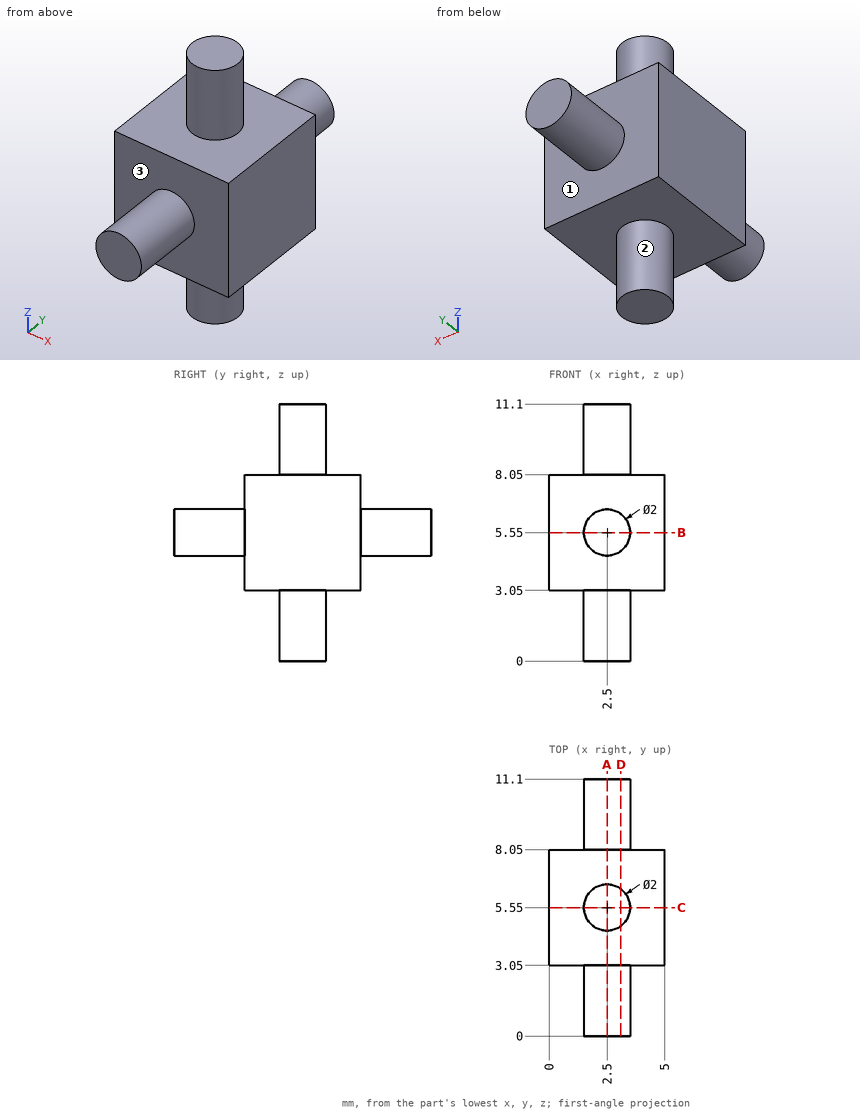
Drawing for the job (mm, zero at the part's lowest x, y, z). A direction names the side the tool comes from. Give positions to 0.01 mm unless a question says otherwise; leave off trailing zeros. Write each loop counter-clockwise with the first axis right and the second up, starting at its lowest first coordinate (ties: lowest second). Pieces come first, ordered by that corner, then holes. Notation, with made-up numbers: M -18,48 L -1,48 A15 cw -1,63 Z; hole C 6.5,42 d2. An arc over 180 degrees is marked long. Return JSON: item names as keys, results as strings. Group by question number.
(1) 3-axis set-ups, long thin cutter, end or side, ignore diameter. For the marked faces 1, 2 and 3: which of +Z, -Z, +X, -X, +Y, -Y reach the whole face in a straight line?
(2) Band-saw the part on B-B (z = 5.55). Give the cut face in (x, y).
(3) Band-saw the part on D-D (x = 3.1). Give the cut face in (y, z), and give its area (3 significant figures).
(4) Flat gauge pins, fed straight in: pin 1 Ø2.5 at (x, z) = (2, 5.5) entering from -Y; pin 2 Ø1 at (y, z) = (9, 2.5) entering from +X. Where does each tip first touch, or does it go through?
(5) Drill centre lines: L1, parallel to Y at x = 2.75, z = 7.75; L2, parallel to Z at x = 2.55, y = 1.75. Where is each one in solid material? Low to high. Write a range as [from, to].
(6) Band-saw the part on A-A (x = 2.5). Give the cut face in (y, z), and give its area (3 significant figures).
Entries:
{
 "1": {"face 1": "+Y", "face 2": "-Z", "face 3": "-Y"},
 "2": {"outline": "M 0,3.05 L 1.5,3.05 L 1.5,0 L 3.5,0 L 3.5,3.05 L 5,3.05 L 5,8.05 L 3.5,8.05 L 3.5,11.1 L 1.5,11.1 L 1.5,8.05 L 0,8.05 Z"},
 "3": {"outline": "M 0,4.75 L 3.05,4.75 L 3.05,3.05 L 4.75,3.05 L 4.75,0 L 6.35,0 L 6.35,3.05 L 8.05,3.05 L 8.05,4.75 L 11.1,4.75 L 11.1,6.35 L 8.05,6.35 L 8.05,8.05 L 6.35,8.05 L 6.35,11.1 L 4.75,11.1 L 4.75,8.05 L 3.05,8.05 L 3.05,6.35 L 0,6.35 Z", "area": "44.5 mm^2"},
 "4": {"pin 1": "stops at y = 0", "pin 2": "passes through"},
 "5": {"L1": "y = [3.05, 8.05]", "L2": "z = [4.55, 6.55]"},
 "6": {"outline": "M 0,4.55 L 3.05,4.55 L 3.05,3.05 L 4.55,3.05 L 4.55,0 L 6.55,0 L 6.55,3.05 L 8.05,3.05 L 8.05,4.55 L 11.1,4.55 L 11.1,6.55 L 8.05,6.55 L 8.05,8.05 L 6.55,8.05 L 6.55,11.1 L 4.55,11.1 L 4.55,8.05 L 3.05,8.05 L 3.05,6.55 L 0,6.55 Z", "area": "49.4 mm^2"}
}
